```python
from build123d import *

# Parameters (mm, degrees)
SALIENTE_EXTRUIR1_DEPTH = 15
CROQUIS4_W              = 2
CROQUIS4_H              = 6
SALIENTE_EXTRUIR2_DEPTH = 15
CROQUIS5_R              = 2.575
CORTAR_EXTRUIR1_DEPTH   = 4


with BuildPart() as part:
    # Croquis2 → Saliente-Extruir1 (new body)
    with BuildSketch(Plane(origin=(0, 0, 0), x_dir=(0, 0, -1), z_dir=(1, 0, 0))):
        Polygon((0, 0), (13, 0), (13, 9.8), (25.65, 9.8), (25.65, 12.8), (10, 12.8), (10, 3), (0, 3), align=None)
    extrude(amount=SALIENTE_EXTRUIR1_DEPTH)

    # Croquis4 → Saliente-Extruir2 (add, through all)
    with BuildSketch(Plane(origin=(0, 0, 0), x_dir=(0, 0, -1), z_dir=(1, 0, 0))):
        with Locations((26.65, 9.8)):
            Rectangle(CROQUIS4_W, CROQUIS4_H)
    extrude(amount=SALIENTE_EXTRUIR2_DEPTH)

    # Croquis5 → Cortar-Extruir1 (cut, through all)
    with BuildSketch(Plane(origin=(0, 3, 0), x_dir=(1, 0, 0), z_dir=(0, 1, 0))):
        with Locations((7.5, 5)):
            Circle(CROQUIS5_R)
    extrude(amount=-CORTAR_EXTRUIR1_DEPTH, mode=Mode.SUBTRACT)


solid = part.part
```
Source: CAD feature listing. Evaluate the final solid. Frame: model axes, mm. A direction names the side the tool comes from. Coordinates: 2 decimals unless noted, no trailing zeros. Write each loop counter-clockwise with the first axis right and the second up, starting at its lowest first coordinate (ties: lowest second). Pieces come first, ordered by that corner, then holes. Notation, with made-up numbers: M 65.5,57.25 L 117.5,57.25 A21 cw 117.5,64.25 Z; hole C 79.25,78 d6. An arc over 180 degrees is marked long. Answer as a JSON object with one key per item and string values.
1. Access query for faces 5 (the flat face through (7, 6.8, -27)), 6 (the flat face through (5.7, 3, -2.8)), 7 (the flat face through (7, 9.8, -19)), 8 (the cylindrical face through (9.879, 1.521, -4.014)). Directions: +Z, -Z, +X, -X, +Y, -Y. A direction counts if a zero-diameter tool reaches every point of the face in a straight line with its end or side. Return the directions, or none.
Evaluation:
{"face 5": "-Z, +X, -X, -Y", "face 6": "+Z, +X, -X, +Y", "face 7": "+X, -X, -Y", "face 8": "+Y, -Y"}
2. Contact query for flat-ended pins moving along their axis: P1, Ø4, axis at x = 7.5, z = -5, coming from the -Y side; P2, Ø2, axis at x = 9, z = -26.5, coming from the -Y side; P3, Ø8, axis at x = 2.5, z = -18.5, coming from the -Y side; P4, Ø1.5, axis at x = 7, y = 8.5, coming from the +Z side. Output: stop coordinate, or through.
Evaluation:
{"P1": "through", "P2": "y = 6.8", "P3": "y = 9.8", "P4": "z = -10"}
3. Cut plane D-D on y = 1.5. Output: boundary loops of the cut face in (x, z) (3 decimals), plus the area to 3 significant figures.
Evaluation:
{"outline": "M 0,-13 L 15,-13 L 15,0 L 0,0 Z; hole C 7.5,-5 d5.15", "area": "174 mm^2"}
4. Draft query along Z for faces 1 (the flat face through (7, 8, -10)), 2 (the flat face through (7, 8, -25.65)), 3 (the flat face through (7, 5, -13)), 4 (the flat face through (15, 6.9, -12.7)). Return one class per face: released by +Z, released by -Z, zero draft, split by the parting line, or undercut.
Evaluation:
{"face 1": "released by +Z", "face 2": "undercut", "face 3": "undercut", "face 4": "zero draft"}
5. Cut plane A-A on z = -5. Output: boundary loops of the cut face in (x, y) (3 decimals).
Evaluation:
{"outline": "M 0,0 L 4.925,0 L 4.925,3 L 0,3 Z; M 10.075,0 L 15,0 L 15,3 L 10.075,3 Z"}
6. Cut plane C-C on x = 7.5. Output: boundary loops of the cut face in (y, z) (3 decimals).
Evaluation:
{"outline": "M 0,-13 L 9.8,-13 L 9.8,-25.65 L 6.8,-25.65 L 6.8,-27.65 L 12.8,-27.65 L 12.8,-10 L 3,-10 L 3,-7.575 L 0,-7.575 Z; M 0,-2.425 L 3,-2.425 L 3,0 L 0,0 Z"}
7. Ray query, L1, parallel to Z at x = 7.75, y = 7.25; L2, parallel to X at y = 2.4, z = -5 (3 decimals); L3, parallel to Z at x = 7.5, y = 1.1 (3 decimals). Return the intervals inside material, ascending.
Evaluation:
{"L1": "-27.65 to -25.65, -13 to -10", "L2": "0 to 4.925, 10.075 to 15", "L3": "-13 to -7.575, -2.425 to 0"}
8. Cut plane B-B on y = 7.5. Output: boundary loops of the cut face in (x, z), plus the area to 3 significant figures.
Evaluation:
{"outline": "M 0,-27.65 L 15,-27.65 L 15,-25.65 L 0,-25.65 Z; M 0,-13 L 15,-13 L 15,-10 L 0,-10 Z", "area": "75.0 mm^2"}
